Input: part model. Units: mm. Frame: model coordinates. Face numbers are marked on the shaded views. A direction names the side the tool comes from. Coordinates: 2 decimals unless noted, no trailing zeros. Write each loop counter-clockwise with the first axis right and the second up, starting at its lowest first coordinate (ties: lowest second). Pieces come first, ordered by that corner, then holes. Notation, with made-up numbers: (53.25, 87) -> (65.25, 87) arc R13 ccw to (65.25, 103) -> close; hole circle Ø3 at (9.25, 42). An arc over 180 degrees is marked (long way). Use one line per item in the form item = value. Start each with the question number.
(1) First-contact query: pin 1 (5 mm diameter, centred on y = 5.5, z = 66, fed in from +X); pin 2 (5 mm diameter, centred on x = -4.5, z = -2.5, fed in from -Y); pin 3 (0.9 mm diameter, centred on x = -14, y = 0.5, fed in from -Z). Flat tips, straight axial feed; report the tip coordinate or a pass-through.
(2) Ray query, line 1 along Z through (x, y) = (-2, 11.5); line 2 along Y through (x, z) = (0, 77). Return the intervals inside material, ascending.
(3) Cut plane A-A on z = 26.5. Return the cut outline in (x, y), plus the area to 3 significant figures.
(4) Pull-direction query (Y, two-part tool) for the marked faces 1, 2 and 3; classes: released by +Y, released by -Y, zero draft, split by the parting line, or undercut.
(5) Cut plane C-C on x = 0. Return the cut outline in (y, z).
(6) Set-up query: the marked faces 4 and 5. Return all of +Z, -Z, +X, -X, +Y, -Y with unobstructed straight access to the full face (end or side cutting, diameter ignored); none if empty.
(7) Cut plane B-B on y = 0. Return the cut outline in (x, z), plus the area to 3 significant figures.
(8) Cut plane D-D on z = 50. Return the cut outline in (x, y), plus the area to 3 significant figures.
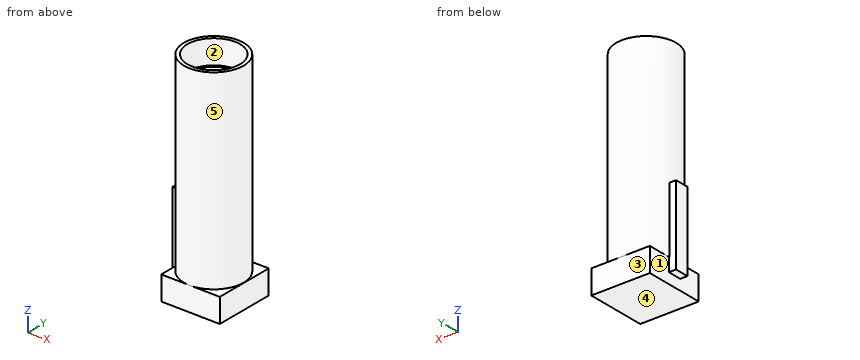
```python
from build123d import *

# Parameters (mm, degrees)
SKETCH_R        = 12.5
PAD_DEPTH       = 80
SKETCH001_R     = 11
POCKET_DEPTH    = 10
SKETCH002_R     = 10
POCKET001_DEPTH = 70.001
SKETCH003_W     = 5
SKETCH003_H     = 2
POCKET002_DEPTH = 70
SKETCH004_W     = 24.485672
SKETCH004_H     = 25.205176
PAD001_DEPTH    = 10
SKETCH005_W     = 5.898827
SKETCH005_H     = 32.91927
PAD002_DEPTH    = 3


with BuildPart() as part:
    # Sketch → Pad (new body)
    with BuildSketch(Plane.XY):
        Circle(SKETCH_R)
    extrude(amount=PAD_DEPTH)

    # Sketch001 (on Face3 of Pad) → Pocket (cut)
    with BuildSketch(Plane.XY.offset(80)):
        Circle(SKETCH001_R)
    extrude(amount=-POCKET_DEPTH, mode=Mode.SUBTRACT)

    # Sketch002 (on Face5 of Pocket) → Pocket001 (cut, through all)
    with BuildSketch(Plane.XY.offset(70)):
        Circle(SKETCH002_R)
    extrude(amount=-POCKET001_DEPTH, mode=Mode.SUBTRACT)

    # Sketch003 (on Face2 of Pocket001) → Pocket002 (cut)
    with BuildSketch(Plane(origin=(0, 0, 0), x_dir=(1, 0, 0), z_dir=(0, 0, -1))):
        with Locations((0, -10.651299)):
            Rectangle(SKETCH003_W, SKETCH003_H)
    extrude(amount=-POCKET002_DEPTH, mode=Mode.SUBTRACT)

    # Sketch004 (on Face2 of Pocket002) → Pad001 (join)
    with BuildSketch(Plane(origin=(0, 0, 0), x_dir=(1, 0, 0), z_dir=(0, 0, -1))):
        with Locations((0.385492, -0.153396)):
            Rectangle(SKETCH004_W, SKETCH004_H)
    extrude(amount=PAD001_DEPTH)

    # Sketch005 (on Face7 of Pad001) → Pad002 (join)
    with BuildSketch(Plane(origin=(-11.857344, 0, 0), x_dir=(0, -1, 0), z_dir=(-1, 0, 0))):
        with Locations((0.006047, 10.84297)):
            Rectangle(SKETCH005_W, SKETCH005_H)
    extrude(amount=PAD002_DEPTH)


solid = part.part
```
Values:
q1.pin_1 = 12.13
q1.pin_2 = -12.45
q1.pin_3 = -5.62
q2.line_1 = -10 to 0, 70 to 80
q2.line_2 = -12.5 to -11, 11 to 12.5
q3.outline = (-14.86, -2.96) -> (-12.15, -2.96) arc R12.5 ccw (long way) to (-12.15, 2.94) -> (-14.86, 2.94) -> close; hole (-2.5, 9.68) arc R10 ccw (long way) to (2.5, 9.68) -> (2.5, 11.65) -> (-2.5, 11.65) -> close
q3.area = 183 mm2
q4.face_1 = zero draft
q4.face_2 = undercut
q4.face_3 = released by +Y
q5.outline = (-12.5, 0) -> (-12.45, 0) -> (-12.45, -10) -> (12.76, -10) -> (12.76, 0) -> (12.5, 0) -> (12.5, 80) -> (11, 80) -> (11, 70) -> (11.65, 70) -> (11.65, 0) -> (-10, 0) -> (-10, 70) -> (-11, 70) -> (-11, 80) -> (-12.5, 80) -> close
q6.face_4 = -Z, +X, -X, +Y, -Y
q6.face_5 = +Z
q7.outline = (-14.86, -5.62) -> (-11.86, -5.62) -> (-11.86, -10) -> (12.63, -10) -> (12.63, 0) -> (12.5, 0) -> (12.5, 80) -> (11, 80) -> (11, 70) -> (10, 70) -> (10, 0) -> (-10, 0) -> (-10, 70) -> (-11, 70) -> (-11, 80) -> (-12.5, 80) -> (-12.5, 27.3) -> (-14.86, 27.3) -> close
q7.area = 706 mm2
q8.outline = circle Ø25 at (0, 0); hole (-2.5, 9.68) arc R10 ccw (long way) to (2.5, 9.68) -> (2.5, 11.65) -> (-2.5, 11.65) -> close
q8.area = 168 mm2
